The figure shows three views and two pictorial views of one solid part (mm, origin at its lowest corner). Answer the questions. A direction names the side the tool comes from. Coordinates: 2 decimals unless noted, no trailing zeros. Write each loop counter-clockwise with the first axis right and the second up, starting at its lowest first coordinate (ties: lowest second). Pieces come first, ordered by that corner, then holes. Notation, with made-up numbers: M 38,-35 L 69,-35 A10 ccw 69,-21 Z; hole C -38.75,33 d5. An arc over 180 degrees is marked long. Use a Markdown table: item, result. Add a question column.
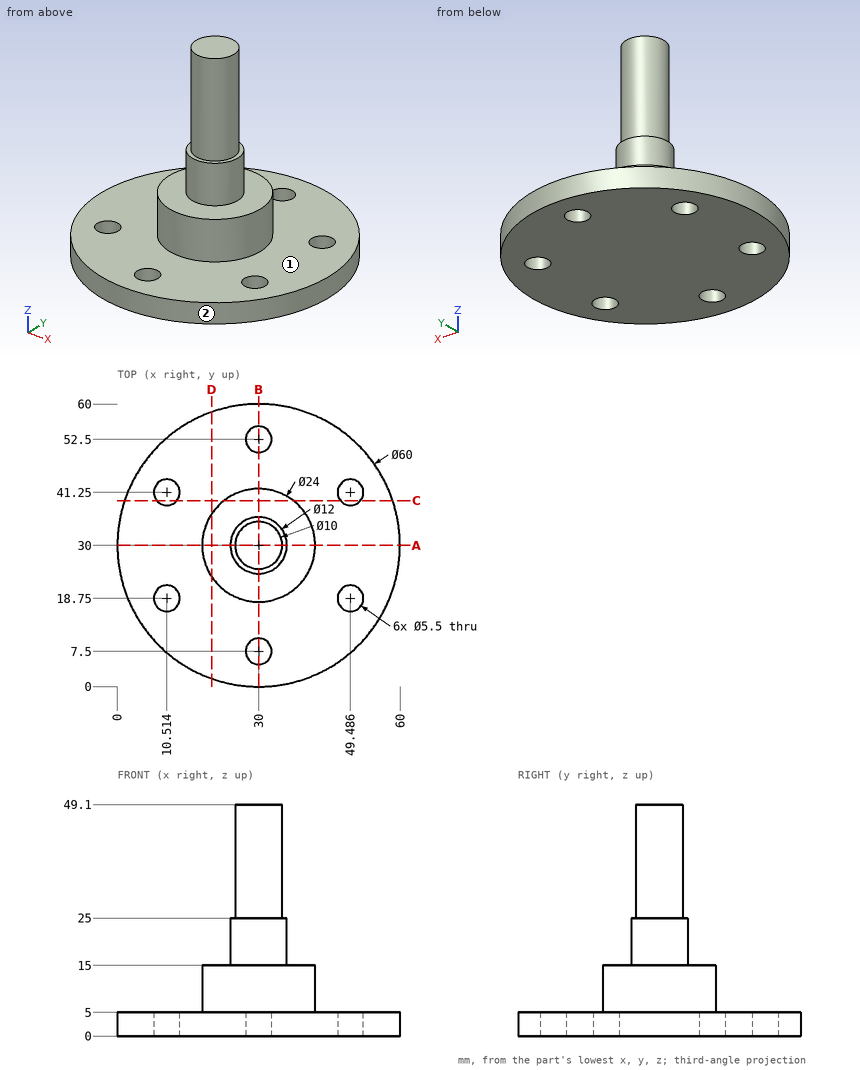
Item 1: For the marked faces 1 and 2, determine the directions among +Z, -Z, +X, -X, +Y, -Y from which every point of the face is accessible in a straight line to the end or side of a thin tool.
Item 2: Consider probe 1 along Y at (x, z) = (30, 1.7); probe 2 along X at (y, z) = (18, 2) (1 decimal); probe 3 along X at (y, z) = (41, 1) (1 decimal). Determine where each line is inside the solid, lowest interval first.
Item 3: Find section A-A on y = 30. Give the vertices of the cut face in (x, z).
Item 4: Find section D-D on x = 20. Give the vertices of the cut face in (y, z) (1 decimal).
Item 5: Find section B-B on x = 30. Give the vertices of the cut face in (y, z).
Item 6: Each of these flat-tipped pins is pushed along its axis until it touches: pin 1 (4 mm diameter, centred on y = 36, z = 20, fed in from +X); pin 2 (5 mm diameter, centred on y = 37.5, z = 25, fed in from +X) (1 decimal); pin 3 (4 mm diameter, centred on x = 7.5, y = 15.5, fed in from +Z). Where does it stop, or does it pass through?
Item 7: Find section C-C on y = 39.5. Give the vertices of the cut face in (x, z) (1 decimal).
Geometry says:
| question | item | result |
|---|---|---|
| 1 | face 1 | +Z |
| 1 | face 2 | +Z, -Z |
| 2 | probe 1 | y = 0 to 4.75, 10.25 to 49.75, 55.25 to 60 |
| 2 | probe 2 | x = 2.5 to 7.9, 13.2 to 46.8, 52.1 to 57.5 |
| 2 | probe 3 | x = 2.1 to 7.8, 13.3 to 46.7, 52.2 to 57.9 |
| 3 | outline | M 0,0 L 60,0 L 60,5 L 42,5 L 42,15 L 36,15 L 36,25 L 35,25 L 35,49.1 L 25,49.1 L 25,25 L 24,25 L 24,15 L 18,15 L 18,5 L 0,5 Z |
| 4 | outline | M 1.7,0 L 58.3,0 L 58.3,5 L 36.6,5 L 36.6,15 L 23.4,15 L 23.4,5 L 1.7,5 Z |
| 5 | outline | M 0,0 L 4.75,0 L 4.75,5 L 0,5 Z; M 10.25,0 L 49.75,0 L 49.75,5 L 42,5 L 42,15 L 36,15 L 36,25 L 35,25 L 35,49.1 L 25,49.1 L 25,25 L 24,25 L 24,15 L 18,15 L 18,5 L 10.25,5 Z; M 55.25,0 L 60,0 L 60,5 L 55.25,5 Z |
| 6 | pin 1 | stops at x = 34.47 |
| 6 | pin 2 | stops at x = 33.3 |
| 6 | pin 3 | stops at z = 5 |
| 7 | outline | M 1.5,0 L 8.4,0 L 8.4,5 L 1.5,5 Z; M 12.6,0 L 47.4,0 L 47.4,5 L 37.3,5 L 37.3,15 L 22.7,15 L 22.7,5 L 12.6,5 Z; M 51.6,0 L 58.5,0 L 58.5,5 L 51.6,5 Z |
